Work out the finished part from the listing and answer in its coordinate system (mm). A direction names the side the tool comes from. Coordinates: 2 decimals unless noted, no trailing zeros. Write each loop counter-clockwise with the first axis right and the second up, starting at its lowest first coordinate (ties: lowest second). Pieces come first, ordered by that corner, then holes. Notation, with made-up numbers: (-20, 13) -> (10, 13) arc R24 cw to (10, 27) -> close; hole circle Ø6 at (15.5, 85.25). An arc over 180 degrees is marked (long way). Write each question's results on one line, items separated by ' | '. Start each with the question number.
from build123d import *

# Parameters (mm, degrees)
F0_R     = 9.525
F1_DEPTH = 6.35
F2_R     = 19.05
F2_R_2   = 9.525
F3_DEPTH = 19.05
F4_W     = 12.7
F4_H     = 38.1
F5_DEPTH = 25.4


with BuildPart() as f1:
    # F0 (on Top) → F1 (new body, symmetric)
    with BuildSketch(Plane.XY):
        with BuildLine():
            ThreePointArc((-6.35, 0), (-11.929616, 13.470384), (-25.4, 19.05))
            ThreePointArc((-25.4, 19.05), (-44.45, 0), (-25.4, -19.05))
            ThreePointArc((-25.4, -19.05), (-11.929616, -13.470384), (-6.35, 0))
        make_face()
        with Locations((-25.4, 0)):
            Circle(F0_R, mode=Mode.SUBTRACT)
        with BuildLine():
            Line((25.4, 19.05), (-25.4, 19.05))
            ThreePointArc((-25.4, 19.05), (-11.929616, 13.470384), (-6.35, 0))
            ThreePointArc((-6.35, 0), (-11.929616, -13.470384), (-25.4, -19.05))
            Line((-25.4, -19.05), (25.4, -19.05))
            Line((25.4, -19.05), (25.4, 19.05))
        make_face()
    extrude(amount=F1_DEPTH, both=True)

    # F2 (on Top) → F3 (join, symmetric)
    with BuildSketch(Plane.XY):
        with Locations((-25.4, 0)):
            Circle(F2_R)
        with Locations((-25.4, 0)):
            Circle(F2_R_2, mode=Mode.SUBTRACT)
    extrude(amount=F3_DEPTH, both=True)

    # F4 (on face) → F5 (join)
    with BuildSketch(Plane.XY.offset(6.35)):
        with Locations((31.75, 0)):
            Rectangle(F4_W, F4_H)
    extrude(amount=-F5_DEPTH)


solid = f1.part
1. For faces 1 (the face through (25.4, 0, -13)), 2 (the face through (-16.6, -3.65, -0.27)), 3 (the face through (-44.43, 0.84, 0.27)), determine the directions among +Z, -Z, +X, -X, +Y, -Y from which every point of the face is accessible in a straight line to the end or side of a thin tool.
2. Find section A-A on z = -16. Give the vertices of the cut face in (x, y) (3 decimals).
3. Find section B-B on y = 0. Give the vertices of the cut face in (x, z) (3 decimals).
4. Find section D-D on z = 16. Give the vertices of the cut face in (x, y) (3 decimals), and give its area (3 significant figures).
5. Given pin 1 Ø10 at (y, z) = (-2, 14) entering from -X; pin 2 Ø6 at (x, y) = (5.5, 12) entering from +Z; pin 3 Ø12 at (y, z) = (12, 10.5) entering from -X, each flat-ended and moving along its own axis, determine where each tip first touches the part or whether it passes through.
6. Find the intervals of material crossed by L1, parallel to Y at x = -25, z = 7; L2, parallel to Z at x = 8.5, y = -8; L3, parallel to X at y = -3, z = -8.5, in increasing order.
7. Find section C-C on x = -29. Give the vertices of the cut face in (y, z), and give its area (3 significant figures).
Ans:
1) face 1: -Z, +Y, -Y | face 2: +Z, -Z | face 3: none
2) outline: circle Ø38.1 at (-25.4, 0); (25.4, -19.05) -> (38.1, -19.05) -> (38.1, 19.05) -> (25.4, 19.05) -> close; hole circle Ø19.05 at (-25.4, 0)
3) outline: (-44.45, -19.05) -> (-34.925, -19.05) -> (-34.925, 19.05) -> (-44.45, 19.05) -> close; (-15.875, -19.05) -> (-6.35, -19.05) -> (-6.35, -6.35) -> (25.4, -6.35) -> (25.4, -19.05) -> (38.1, -19.05) -> (38.1, 6.35) -> (-6.35, 6.35) -> (-6.35, 19.05) -> (-15.875, 19.05) -> close
4) outline: circle Ø38.1 at (-25.4, 0); hole circle Ø19.05 at (-25.4, 0) | area: 855 mm²
5) pin 1: stops at x = -44.45 | pin 2: stops at z = 6.35 | pin 3: stops at x = -43.48
6) L1: y = -19.05 to -9.52, 9.52 to 19.05 | L2: z = -6.35 to 6.35 | L3: x = -44.21 to -34.44, -16.36 to -6.59, 25.4 to 38.1
7) outline: (-18.71, -19.05) -> (-8.82, -19.05) -> (-8.82, 19.05) -> (-18.71, 19.05) -> close; (8.82, -19.05) -> (18.71, -19.05) -> (18.71, 19.05) -> (8.82, 19.05) -> close | area: 753 mm²
